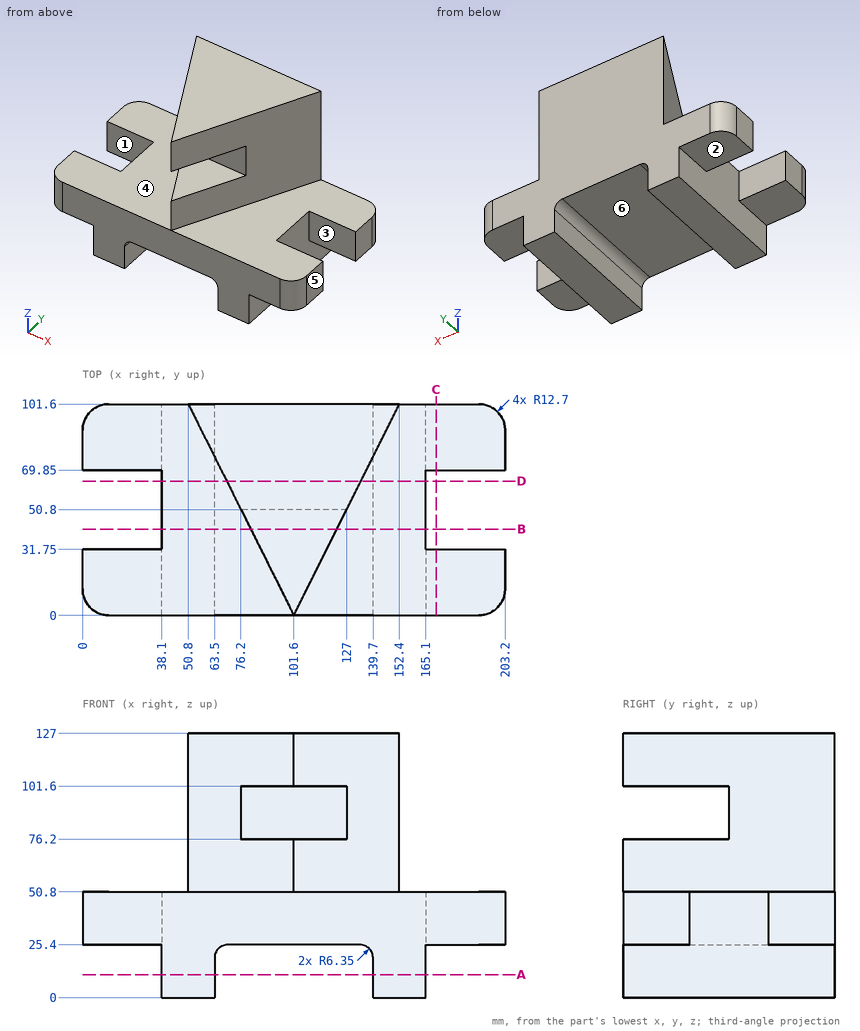
Study the drawing (mm; zero at the part's minimum x, y, z) and answer. A direction names the side the tool comes from. Give positions to 0.01 mm unless a question says otherwise; leave off trailing zeros. Loops run counter-clockwise (first coordinate to the right, second up) from the corner with the lowest first, then second, coordinate; pieces in that order, holes last. Notation, with made-up numbers: (-22.5, 53.5) -> (34.5, 53.5) arc R23 cw to (34.5, 85.5) -> close; hole circle Ø9 at (85, -5.5). An arc over 180 degrees is marked (long way). Write item = value, one per line. Start each with the question number.
(1) Which of the six approach directions +Z, -Z, +X, -X, +Y, -Y give full straight-line access (tool end or side, diameter ignored) to the marked faces 1, 2 and 3?
(2) Find section C-C on x = 170. Give the vertices of the cut face in (y, z).
(3) Find section A-A on z = 11. Give the vertices of the cut face in (x, y), and give its area (3 significant figures).
(4) Given pin 1 Ø4 at (x, y) = (49.5, 30.5) entering from -Z; pin 2 Ø21 at (y, z) = (43, 14) entering from -X; pin 3 Ø1.5 at (x, y) = (155, 17.5) entering from +Z; pin 4 Ø15 at (y, z) = (28, 10) entering from +X, each flat-ended and moving along its own axis, determine where each tip first touches the part or whether it passes through.
(5) Find section D-D on y = 64.5. Give the vertices of the cut face in (x, z).
(6) Find section B-B on y = 41.5. Give the vertices of the cut face in (x, z).
(7) The mould has two halves that part along X. Classify the marked faces 4, 5 and 6: +X half, -X half, draft (parallel to the pull), parting line (faces both ways), or undercut.
(8) Find the intervals of material crossed by probe 1 along X at (y, z) = (39, 8.5); probe 2 along Z at (x, y) = (145, 38); probe 3 along Z at (x, y) = (172, 8), in increasing order. Write a range as from..to.
From the geometry:
q1.face_1 = +Z, -Z, -X
q1.face_2 = -Z, -X, +Y, -Y
q1.face_3 = +Z, -Z, +X
q2.outline = (0, 25.4) -> (31.75, 25.4) -> (31.75, 50.8) -> (0, 50.8) -> close; (69.85, 25.4) -> (101.6, 25.4) -> (101.6, 50.8) -> (69.85, 50.8) -> close
q3.outline = (38.1, 0) -> (63.5, 0) -> (63.5, 101.6) -> (38.1, 101.6) -> close; (139.7, 0) -> (165.1, 0) -> (165.1, 101.6) -> (139.7, 101.6) -> close
q3.area = 5,160 mm^2
q4.pin_1 = 0
q4.pin_2 = 38.1
q4.pin_3 = 50.8
q4.pin_4 = 165.1
q5.outline = (38.1, 0) -> (63.5, 0) -> (63.5, 19.05) arc R6.35 cw to (69.85, 25.4) -> (133.35, 25.4) arc R6.35 cw to (139.7, 19.05) -> (139.7, 0) -> (165.1, 0) -> (165.1, 50.8) -> (133.85, 50.8) -> (133.85, 127) -> (69.35, 127) -> (69.35, 50.8) -> (38.1, 50.8) -> close
q6.outline = (38.1, 0) -> (63.5, 0) -> (63.5, 19.05) arc R6.35 cw to (69.85, 25.4) -> (133.35, 25.4) arc R6.35 cw to (139.7, 19.05) -> (139.7, 0) -> (165.1, 0) -> (165.1, 50.8) -> (122.35, 50.8) -> (122.35, 76.2) -> (80.85, 76.2) -> (80.85, 50.8) -> (38.1, 50.8) -> close; (80.85, 101.6) -> (122.35, 101.6) -> (122.35, 127) -> (80.85, 127) -> close
q7.face_4 = draft
q7.face_5 = +X half
q7.face_6 = undercut
q8.probe_1 = 38.1..63.5, 139.7..165.1
q8.probe_2 = 0..50.8
q8.probe_3 = 25.4..50.8
